```python
from build123d import *

# Parameters (mm, degrees)
SKETCH_1_W      = 22.5
SKETCH_1_H      = 17
EXTRUDE_1_DEPTH = 3
HOLE_WIZARD_1_D = 2.3
SKETCH_5_W      = 22.5
SKETCH_5_H      = 30
EXTRUDE_2_DEPTH = 3
SKETCH_6_W      = 17.5
SKETCH_6_H      = 20
EXTRUDE_3_DEPTH = 3
HOLE_WIZARD_2_D = 3.3
HOLE_WIZARD_3_D = 3


with BuildPart() as part:
    # 草图1 → 凸台-拉伸1 (new body)
    with BuildSketch(Plane(origin=(0, 0, 0), x_dir=(1, 0, 0), z_dir=(0, 1, 0))):
        Rectangle(SKETCH_1_W, SKETCH_1_H)
    extrude(amount=EXTRUDE_1_DEPTH)

    # 孔1 (through all)
    with Locations(Plane(origin=(0, 3, 0), x_dir=(1, 0, 0), z_dir=(0, 1, 0))):
        with Locations((-4, 6), (4, 6), (-4, -6), (4, -6)):
            Hole(HOLE_WIZARD_1_D / 2)

    # 草图5 → 凸台-拉伸2 (add)
    with BuildSketch(Plane(origin=(0, 3, 0), x_dir=(1, 0, 0), z_dir=(0, 1, 0))):
        with Locations((0, -23.5)):
            Rectangle(SKETCH_5_W, SKETCH_5_H)
    extrude(amount=-EXTRUDE_2_DEPTH)

    # 草图6 → 凸台-拉伸3 (add)
    with BuildSketch(Plane(origin=(0, 3, 0), x_dir=(1, 0, 0), z_dir=(0, 1, 0))):
        with Locations((-20, -28.5)):
            Rectangle(SKETCH_6_W, SKETCH_6_H)
    extrude(amount=-EXTRUDE_3_DEPTH)

    # 孔2 (through all)
    with Locations(Plane(origin=(0, 3, 0), x_dir=(1, 0, 0), z_dir=(0, 1, 0))):
        with Locations((6.25, -34.5), (6.25, -54.5), (-13.75, -54.5), (-13.75, -34.5)):
            Hole(HOLE_WIZARD_2_D / 2)

    # 孔3 (through all)
    with Locations(Plane(origin=(0, 3, 0), x_dir=(1, 0, 0), z_dir=(0, 1, 0))):
        with Locations((-12.75, -18.5)):
            Hole(HOLE_WIZARD_3_D / 2)


solid = part.part
```
Can you work these out from the model? Positions are in its coordinate system, mm. A direction names the side the tool comes from. Coordinates: 2 decimals unless noted, no trailing zeros. Loops run counter-clockwise (first coordinate to the right, second up) from the corner with the lowest first, then second, coordinate; pieces in that order, holes last. Notation, with made-up numbers: (-26, -16.5) - (28, -16.5) arc R13 ccw to (28, -1.5) - close; hole circle Ø3 at (8.25, -18). An arc over 180 degrees is marked (long way). Use a Markdown table: item, result.
Item 1: I want a section at B-B on z = -6. Please give me the cut outline in (x, y), and give its area (3 significant figures).
Numbers:
| item | result |
|---|---|
| outline | (-11.25, 0) - (-5.15, 0) - (-5.15, 3) - (-11.25, 3) - close; (-2.85, 0) - (2.85, 0) - (2.85, 3) - (-2.85, 3) - close; (5.15, 0) - (11.25, 0) - (11.25, 3) - (5.15, 3) - close |
| area | 53.7 mm2 |
Item 2: We'd pull the mould along X, two halves only. Please class faces 3 (the face through (11.25, 2, 15)), 4 (the face through (-5, 0, 20)), 5 (the face through (-3.152, 1.479, -6.777)): released by +X, released by -X, zero draft, split by the parting line, or undercut.
Numbers:
| item | result |
|---|---|
| face 3 | released by +X |
| face 4 | zero draft |
| face 5 | undercut |
Item 3: I want a section at A-A on x = 6.25. Please give me the cut outline in (y, z).
Numbers:
| item | result |
|---|---|
| outline | (0, -8.5) - (3, -8.5) - (3, 32.85) - (0, 32.85) - close; (0, 36.15) - (3, 36.15) - (3, 38.5) - (0, 38.5) - close |
Item 4: If I drill on probe 1 along Z at (x, y) = (4, 0.8); probe 2 along X at (y, z) = (1.1, 34.5); probe 3 along X at (y, z) = (1.25, 6), over which ranges is the centre line in solid material (lowest first)? Write a range as from..to.
Numbers:
| item | result |
|---|---|
| probe 1 | z = -8.5..-7.15, -4.85..4.85, 7.15..38.5 |
| probe 2 | x = -28.75..-15.4, -12.1..4.6, 7.9..11.25 |
| probe 3 | x = -11.25..-5.15, -2.85..2.85, 5.15..11.25 |
Item 5: For faces 1 (the face through (-9, 2, 38.5)), 2 (the face through (-22, 2, 18.5)), which set-ups out of +Z, -Z, +X, -X, +Y, -Y let a thin tool reach every point of the face, with its end or its side?
Numbers:
| item | result |
|---|---|
| face 1 | +Z, +X, -X, +Y, -Y |
| face 2 | -Z, -X, +Y, -Y |
Item 6: I want a section at C-C on y = 1.8. Please give me the cut outline in (x, z), and give its area (3 significant figures).
Numbers:
| item | result |
|---|---|
| outline | (-28.75, 18.5) - (-14.25, 18.5) arc R1.5 cw to (-11.25, 18.5) - (-11.25, -8.5) - (11.25, -8.5) - (11.25, 38.5) - (-28.75, 38.5) - close; hole circle Ø3.3 at (-13.75, 34.5); hole circle Ø2.3 at (-4, -6); hole circle Ø2.3 at (-4, 6); hole circle Ø2.3 at (4, -6); hole circle Ø2.3 at (4, 6); hole circle Ø3.3 at (6.25, 34.5) |
| area | 1,370 mm2 |
Item 7: Will these pins go through, and if not, where does the flat tip stop? pin 1 (2 mm diameter, centred on x = 4, z = 6, fed in from +Y); pin 2 (1.5 mm diameter, centred on y = 1, z = 6, fed in from -X); pin 3 (1.5 mm diameter, centred on x = -24.5, y = 1.5, fed in from -Z).
Numbers:
| item | result |
|---|---|
| pin 1 | passes through |
| pin 2 | stops at x = -11.25 |
| pin 3 | stops at z = 18.5 |
Item 8: I want a section at D-D on x = -4. Please give me the cut outline in (y, z), and give its area (3 significant figures).
Numbers:
| item | result |
|---|---|
| outline | (0, -8.5) - (3, -8.5) - (3, -7.15) - (0, -7.15) - close; (0, -4.85) - (3, -4.85) - (3, 4.85) - (0, 4.85) - close; (0, 7.15) - (3, 7.15) - (3, 38.5) - (0, 38.5) - close |
| area | 127 mm2 |
